from build123d import *

# Parameters (mm, degrees)
DODANIE_WYCI_GNI_CIE1_DEPTH = 25
ZAOKR_GLENIE3_R             = 1


with BuildPart() as part:
    # Szkic1 → Dodanie-wyciągnięcie1 (new body)
    with BuildSketch(Plane.XY):
        Polygon((-34.478406184, 29.894019729), (-34.478406184, -16.105980271), (-24.478406184, -16.105980271), (-24.478406184, -31.105980271), (61.521593816, -31.105980271), (61.521593816, 29.894019729), align=None)
    extrude(amount=DODANIE_WYCI_GNI_CIE1_DEPTH)

    # Zaokrąglenie3
    zaokr_glenie3_edges = [part.edges().sort_by_distance(p)[0] for p in [
        (-29.478406184, -16.105980271, 25),
        (61.521593816, 29.894019729, 12.5),
        (61.521593816, -31.105980271, 12.5),
        (-24.478406184, -31.105980271, 12.5),
        (-24.478406184, -16.105980271, 12.5),
        (-34.478406184, -16.105980271, 12.5),
        (-34.478406184, 29.894019729, 12.5),
        (-24.478406184, -23.605980271, 25),
        (18.521593816, -31.105980271, 25),
        (61.521593816, -0.605980271, 25),
        (13.521593816, 29.894019729, 25),
        (61.521593816, -0.605980271, 0),
        (18.521593816, -31.105980271, 0),
        (-24.478406184, -23.605980271, 0),
        (-34.478406184, 6.894019729, 25),
        (-29.478406184, -16.105980271, 0),
        (-34.478406184, 6.894019729, 0),
        (13.521593816, 29.894019729, 0),
    ]]
    fillet(zaokr_glenie3_edges, radius=ZAOKR_GLENIE3_R)


solid = part.part
Read the model definition and answer for the solid it produces. Units are mm, in the model's axes. A direction names the side the tool comes from. Coordinates: 2 decimals unless noted, no trailing zeros. Loops run counter-clockwise (first coordinate to the right, second up) from the corner with the lowest first, then second, coordinate; pieces in that order, holes last. Notation, with made-up numbers: (70, 42) -> (94, 42) arc R15 cw to (94, 67) -> close; hole circle Ø10 at (12, 34.5). An arc over 180 degrees is marked (long way). Answer in a Markdown table with one row per item.
Item 1: For faces 1 (the flat face through (61.522, -1, 12)), 2 (the flat face through (-24.478, -24, 12)), determine the directions among +Z, -Z, +X, -X, +Y, -Y from which every point of the face is accessible in a straight line to the end or side of a thin tool.
Returned:
| item | result |
|---|---|
| face 1 | +Z, -Z, +X, +Y, -Y |
| face 2 | +Z, -Z, -X, -Y |
Item 2: Straight lines are drawn through the part: line 1 along Y through (x, z) = (-25.5, 8.5); line 2 along X through (y, z) = (-22, 4). For each, find the intervals that lie inside material, in ascending order. Write a range as [from, to].
Returned:
| item | result |
|---|---|
| line 1 | y = [-16.11, 29.89] |
| line 2 | x = [-24.48, 61.52] |
Item 3: A cutting plane is placed at A-A on y = -26. Determine the outline of the cut face in (x, z), plus the area to 3 significant figures.
Returned:
| item | result |
|---|---|
| outline | (-24.48, 1) arc R1 ccw to (-23.48, 0) -> (60.52, 0) arc R1 ccw to (61.52, 1) -> (61.52, 24) arc R1 ccw to (60.52, 25) -> (-23.48, 25) arc R1 ccw to (-24.48, 24) -> close |
| area | 2,150 mm^2 |
Item 4: A cutting plane is placed at B-B on z = 4.5. Determine the outline of the cut face in (x, y).
Returned:
| item | result |
|---|---|
| outline | (-34.48, -15.11) arc R1 ccw to (-33.48, -16.11) -> (-25.48, -16.11) arc R1 cw to (-24.48, -17.11) -> (-24.48, -30.11) arc R1 ccw to (-23.48, -31.11) -> (60.52, -31.11) arc R1 ccw to (61.52, -30.11) -> (61.52, 28.89) arc R1 ccw to (60.52, 29.89) -> (-33.48, 29.89) arc R1 ccw to (-34.48, 28.89) -> close |
Item 5: Each of these flat-tipped pins is pushed along its axis until it touches: P1, Ø14.5, axis at y = -22, z = 14, coming from the -X side; P2, Ø9, axis at x = -31.5, z = 17, coming from the -Y side. Where does it stop, or does it pass through?
Returned:
| item | result |
|---|---|
| P1 | stops at x = -34.48 |
| P2 | stops at y = -16.11 |
